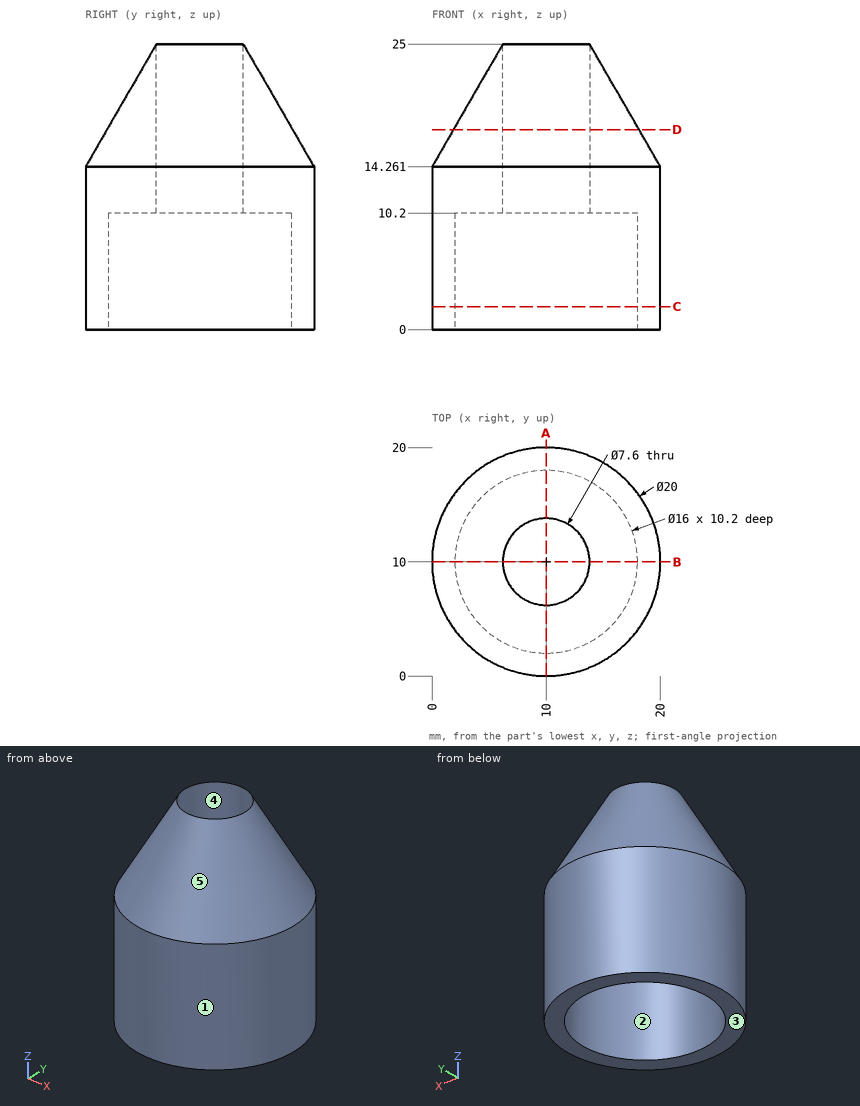
Print and shaded views of the part. All mm, measured from the part's lowest x, y and z. A direction names the side the tool comes from. Round coordinates to 2 decimals unless told otherwise and drop trailing zeros. Write each loop counter-clockwise with the first axis right and the second up, starting at its lowest first coordinate (ties: lowest second). Pieces come first, ordered by that corner, then holes.
(1) Slice it at D-D, the plane z = 17.5. Write the cut outline in (x, y), and give its area (3 significant figures).
(2) Probe line 1 along X through (y, z) = (9.75, 5.25); line 2 along Y through (x, z) = (8.5, 7.5); line 3 along Y through (x, z) = (10.5, 19.5). List the from-to ranges inside material, lowest first.
(3) 3-axis set-ups, long thin cutter, end or side, ignore diameter. For the marked faces 1 and 2: which of +Z, -Z, +X, -X, +Y, -Y reach the whole face in a straight line?
(4) Mould opens along X. For the marked faces 3, 4 and 5 say: pulls with the +X half, pulls with the -X half, needs draft (parallel to the pull), parting line crosses it, or undercut.
(5) Drop flat-ended pins along their axis: P1, Ø6, axis at x = 8.5, y = 7, coming from the -Z side; P2, Ø3, axis at x = 12, z = 12, coming from the -Y side; P3, Ø2, axis at x = 12.5, z = 8.5, coming from the -Y side; P4, Ø6, axis at x = 10, y = 10, coming from the -Z side. Give the stop position or say it passes through.
(6) Slice it at A-A, the plane x = 10. Write the cut outline in (y, z), and give its area (3 significant figures).
(7) Slice it at C-C, the plane z = 2. Write the cut outline in (x, y).
From the geometry:
1. outline: circle Ø16.26 at (10, 10); hole circle Ø7.6 at (10, 10)
1. area: 162 mm2
2. line 1: x = 0 to 2, 18 to 20
2. line 2: y = 0.11 to 2.14, 17.86 to 19.89
2. line 3: y = 3.04 to 6.23, 13.77 to 16.96
3. face 1: +Z, -Z
3. face 2: -Z
4. face 3: needs draft
4. face 4: undercut
4. face 5: parting line crosses it
5. P1: stops at z = 10.2
5. P2: stops at y = 0.01
5. P3: stops at y = 0.11
5. P4: passes through
6. outline: (0, 0) - (2, 0) - (2, 10.2) - (6.2, 10.2) - (6.2, 25) - (0, 14.26) - close; (13.8, 10.2) - (18, 10.2) - (18, 0) - (20, 0) - (20, 14.26) - (13.8, 25) - close
6. area: 158 mm2
7. outline: circle Ø20 at (10, 10); hole circle Ø16 at (10, 10)
